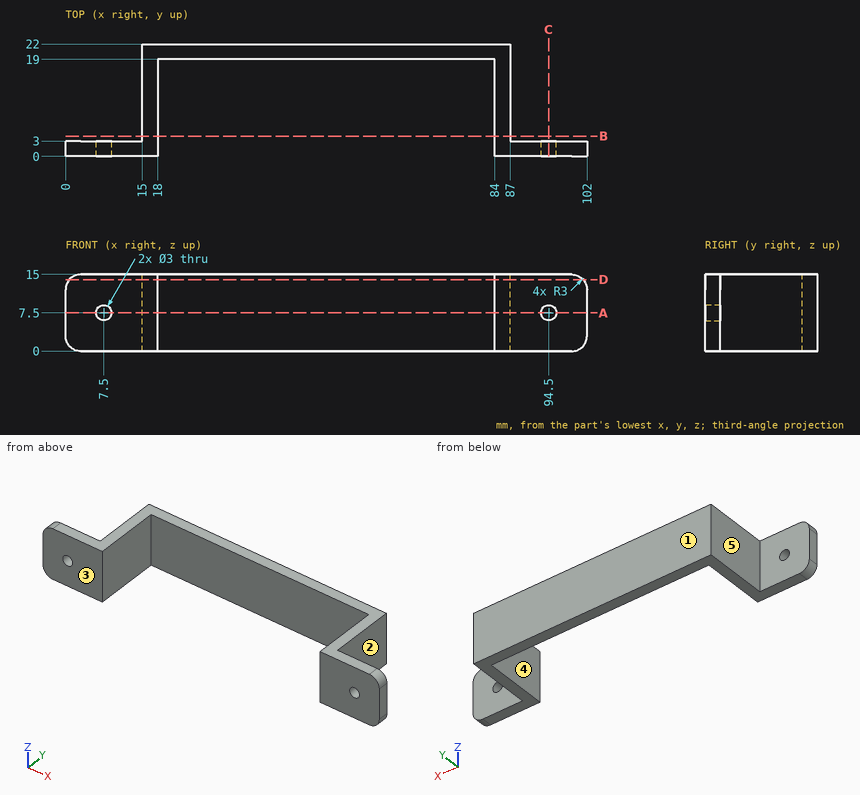
Source: three-view drawing plus pictorial views. Frame: mm from the lowest corner of the part. A direction names the side the tool comes from. Round coordinates to 2 decimals unless told otherwise and drop trailing zeros. Loops run counter-clockwise (first coordinate to the right, second up) from the corner with the lowest first, then second, coordinate; pieces in that order, holes last.
Q1. Section D-D, the plane z = 14. Return loops of the section in (x, y).
Q2. Section A-A, the plane z = 7.5. Return loops of the section in (x, y), plus the area to 3 significant figures.
Q3. Ray query, line 1 (X direction, y = 1.4, z = 7.5); line 2 (Z direction, x = 94.5, y = 1.85); line 3 (X direction, y = 16.25, z = 8). Return the intervals inside material, ascending.
Q4. Section B-B, the plane y = 4. Return loops of the section in (x, z), plus the area to 3 significant figures.
Q5. Access query for the marked faces 1, 2, 3, 4 and 5. Directions: +Z, -Z, +X, -X, +Y, -Y. A direction counts if a zero-diameter tool reaches every point of the face in a straight line with its end or side. Return the directions, or none.
Q6. Section C-C, the plane x = 94.5. Return loops of the section in (y, z), plus the area to 3 significant figures.
Q7. First-contact query: P1, Ø4.5, axis at y = 16.5, z = 7, coming from the -X side; P2, Ø2, axis at x = 69, z = 2.5, coming from the -Y side; P3, Ø7.5, axis at y = 14.5, z = 9.5, coming from the +X side. Flat tips, straight axial feed; report the tip coordinate or a pass-through.
Solutions:
1. outline: (0.76, 0) - (18, 0) - (18, 19) - (84, 19) - (84, 0) - (101.24, 0) - (101.24, 3) - (87, 3) - (87, 22) - (15, 22) - (15, 3) - (0.76, 3) - close
2. outline: (0, 0) - (6, 0) - (6, 3) - (0, 3) - close; (9, 0) - (18, 0) - (18, 19) - (84, 19) - (84, 0) - (93, 0) - (93, 3) - (87, 3) - (87, 22) - (15, 22) - (15, 3) - (9, 3) - close; (96, 0) - (102, 0) - (102, 3) - (96, 3) - close
2. area: 402 mm2
3. line 1: x = 0 to 6, 9 to 18, 84 to 93, 96 to 102
3. line 2: z = 0 to 6, 9 to 15
3. line 3: x = 15 to 18, 84 to 87
4. outline: (15, 0) - (18, 0) - (18, 15) - (15, 15) - close; (84, 0) - (87, 0) - (87, 15) - (84, 15) - close
4. area: 90.0 mm2
5. face 1: +Z, -Z, +X, -X, +Y
5. face 2: +Z, -Z, +X, +Y
5. face 3: +Z, -Z, +X, -X, -Y
5. face 4: +Z, -Z, -Y
5. face 5: +Z, -Z, -X, +Y
6. outline: (0, 0) - (3, 0) - (3, 6) - (0, 6) - close; (0, 9) - (3, 9) - (3, 15) - (0, 15) - close
6. area: 36.0 mm2
7. P1: stops at x = 15
7. P2: stops at y = 19
7. P3: stops at x = 87
